Work out the finished part from the listing and answer in its coordinate system (mm). A direction names the side the tool comes from. Coordinates: 2 decimals unless noted, no trailing zeros. Order: outer loops, then holes, each group sorted by start corner. A loop starts at its lowest first (then second) coordinate and runs counter-clockwise, first axis right, second up. Notation, with made-up numbers: M 0,12.5 L 27,12.5 A29 ccw 27,35.5 Z; hole C 39,3.5 d3. An arc over 180 degrees is marked long. Use a Markdown table: item, result.
from build123d import *

# Parameters (mm, degrees)
F0_W     = 100
F0_H     = 85
F1_DEPTH = 3
F2_R     = 2.9
F3_DEPTH = 7
F2_R_2   = 4
F4_DEPTH = 1


with BuildPart() as f1:
    # F0 (on Top) → F1 (new body)
    with BuildSketch(Plane.XY):
        with Locations((-15.346884, 6.289634)):
            Rectangle(F0_W, F0_H)
    extrude(amount=F1_DEPTH)

    # F2 (on face) → F3 (join)
    with BuildSketch(Plane.XY.offset(3)):
        with Locations((-43.702953, -11.385884)):
            Circle(F2_R)
        with Locations((25.821336, 39.657585)):
            Circle(F2_R)
    extrude(amount=F3_DEPTH)

    # F2 (on face) → F4 (join)
    with BuildSketch(Plane.XY.offset(3)):
        with Locations((-43.702953, -11.385884)):
            Circle(F2_R_2)
        with Locations((-43.702953, -11.385884)):
            Circle(F2_R, mode=Mode.SUBTRACT)
        with Locations((25.821336, 39.657585)):
            Circle(F2_R_2)
        with Locations((25.821336, 39.657585)):
            Circle(F2_R, mode=Mode.SUBTRACT)
    extrude(amount=F4_DEPTH)


solid = f1.part
1. For a pull along Z with two mould halves and no side action, classify faces 1 (the face through (-16, 7, 0)), 2 (the face through (25.444, 42.533, 6.958)), 3 (the face through (-16, 7, 3)) as +Z half, -Z half, draft (parallel to the pull), parting line (faces both ways), or undercut.
Answers below:
| item | result |
|---|---|
| face 1 | -Z half |
| face 2 | draft |
| face 3 | +Z half |
2. Section B-B on z = 8.5 is taken. Determine the outline of the cut face in (x, y).
Answers below:
| item | result |
|---|---|
| outline | C -43.7,-11.39 d5.8; C 25.82,39.66 d5.8 |
3. Section A-A on x = -42 is taken. Determine the outline of the cut face in (y, z), then the cut area to 3 significant figures.
Answers below:
| item | result |
|---|---|
| outline | M -36.21,0 L 48.79,0 L 48.79,3 L -7.77,3 L -7.77,4 L -9.04,4 L -9.04,10 L -13.73,10 L -13.73,4 L -15.01,4 L -15.01,3 L -36.21,3 Z |
| area | 290 mm² |
4. Section C-C on y = 25.5 is taken. Determine the outline of the cut face in (x, z), then the cut area to 3 significant figures.
Answers below:
| item | result |
|---|---|
| outline | M -65.35,0 L 34.65,0 L 34.65,3 L -65.35,3 Z |
| area | 300 mm² |
5. Find the intervals of material crossed by probe 1 along Z at (x, y) = (1, 38.5); probe 2 along X at (y, z) = (41, 9.75), in increasing order.
Answers below:
| item | result |
|---|---|
| probe 1 | 0 to 3 |
| probe 2 | 23.25 to 28.39 |
6. Section D-D on x = 27 is taken. Determine the outline of the cut face in (y, z), then the cut area to 3 significant figures.
Answers below:
| item | result |
|---|---|
| outline | M -36.21,0 L 48.79,0 L 48.79,3 L 43.48,3 L 43.48,4 L 42.31,4 L 42.31,10 L 37.01,10 L 37.01,4 L 35.84,4 L 35.84,3 L -36.21,3 Z |
| area | 294 mm² |
7. A flat-ended cylindrical pin translates along its axis: P1, Ø1.5, axis at x = -17, y = -13, coming from the +Z side. Find the tip coordinate at first contact, or state that the pin passes through.
Answers below:
| item | result |
|---|---|
| P1 | z = 3 |
8. For faces 4 (the face through (28, 42, 4)), 5 (the face through (-65.347, 6, 1)), determine the directions among +Z, -Z, +X, -X, +Y, -Y from which every point of the face is accessible in a straight line to the end or side of a thin tool.
Answers below:
| item | result |
|---|---|
| face 4 | +Z |
| face 5 | +Z, -Z, -X, +Y, -Y |
